Verification items for the finished model (mm, model axes). A direction names the side the tool comes from. Round coordinates to 2 decimals unless told otherwise and drop trailing zeros. Order: outer loops, then holes, each group sorted by start corner. A loop starts at its lowest first (then second) coordinate and runs counter-clockwise, first axis right, second up. Notation, with made-up numbers: M 83.5,0.25 L 123.5,0.25 A19 ccw 123.5,20.25 Z; hole C 29,17 d5. An arc over 180 degrees is marked long. One line per item, written item: value. Start each with the question number.
Autodesk Inventor part; units mm, degrees
ref_plane "YZ Plane" through (0, 0, 0) normal (1, 0, 0) x (0, 1, 0)
ref_plane "XZ Plane" through (0, 0, 0) normal (0, 1, 0) x (-1, 0, 0)
ref_plane "XY Plane" through (0, 0, 0) normal (0, 0, 1) x (1, 0, 0)
sketch "Sketch1" plane through (0, 0, 0) normal (0, 1, 0) x (-1, 0, 0)
  line L0 (-23.3466, 0) -> (-154.4106, 0)
  line L1 (-102.87, 54.61) -> (-74.9238, 54.61)
  line L2 (-88.9, 0) -> (-23.3466, 0)
  line L3 (-88.9, 0) -> (-154.4106, 0)
  arc A0 (-102.87, 54.61) -> (-154.4106, 0) centre (-133.35, 31.75) ccw
  arc A1 (-23.3466, 0) -> (-74.9238, 54.61) centre (-44.4805, 31.7012) ccw
  point P0 (0, 0)
  dimension "d2" = 76.2
  dimension "d3" = 76.2
  dimension "d5" = 131.064
  dimension "d10" = 54.61
extrude "Extrusion1" add sketch "Sketch1" along normal blind 31.75
shell "Shell1" thickness 3.81 removed faces 1 at (84.227, 31.75, 18.2033)
properties part number "paitent remote box"
1. Section check C-C (z = 46). Record the cut outline in (x, y), and give its area (3 significant figures).
2. Tool access check on faces 4 (the face through (89, 16, 54.61)), 5 (the face through (21.212, 17.584, 56.888)), 6 (the face through (17.4, 15.7, 58.5)). Record the directions out of +Z, -Z, +X, -X, +Y, -Y that give a thin tool (end or side, any length) a straight path to the whole face; none if there is none.
3. Depth check by flat-ended pin: pin 1 (1.5 mm diameter, centred on y = 14, z = 50, fed in from -X); pin 2 (8 mm diameter, centred on x = 116, z = 55, fed in from +Y); pin 3 (1 mm diameter, centred on x = 77, y = 4.5, fed in from +Z). Enter the tip coordinate at first touch or a pass-through.
4. Section check A-A (y = 8). Record the cut outline in (x, z).
5. Scan lines: line 1 along X through (y, z) = (10, 58.5); line 2 along Z through (x, y) = (133, 26); line 3 along Z through (x, y) = (96, 8). Record each from-to range of solid material in increasing order.
6. Section check B-B (x = 113). Record the cut outline in (y, z), and give its area (3 significant figures).
7. Draft check along Z on faces 1 (the face through (157.83, 17.58, 55.76)), 2 (the face through (161.688, 15.653, 57.218)), 3 (the face through (83, 31.75, 53)). Enter one of: released by +Z, released by -Z, zero draft, split by the parting line, or undercut.
Geometry check:
1. outline: M 9.17,0 L 168.68,0 L 168.68,31.75 L 164.54,31.75 L 164.54,3.81 L 13.31,3.81 L 13.31,31.75 L 9.17,31.75 Z
1. area: 840 mm²
2. face 4: +Z, +Y, -Y
2. face 5: +Y
2. face 6: +Y, -Y
3. pin 1: stops at x = 10.66
3. pin 2: stops at y = 3.81
3. pin 3: stops at z = 54.61
4. outline: M 23.35,0 L 154.41,0 A38.1 ccw long 102.87,54.61 L 74.92,54.61 A38.1 ccw long Z; hole M 24.53,3.81 L 153.23,3.81 A34.29 ccw long 104.84,50.8 L 72.96,50.8 A34.29 ccw long Z
5. line 1: x = 17.4 to 23.09, 65.87 to 71.56, 106.22 to 111.9, 154.8 to 160.48
5. line 2: z = 0 to 3.81, 66.04 to 69.85
5. line 3: z = 0 to 3.81, 50.8 to 54.61
6. outline: M 0,0 L 31.75,0 L 31.75,3.81 L 3.81,3.81 L 3.81,59.35 L 31.75,59.35 L 31.75,63.96 L 0,63.96 Z
6. area: 479 mm²
7. face 1: undercut
7. face 2: split by the parting line
7. face 3: zero draft
